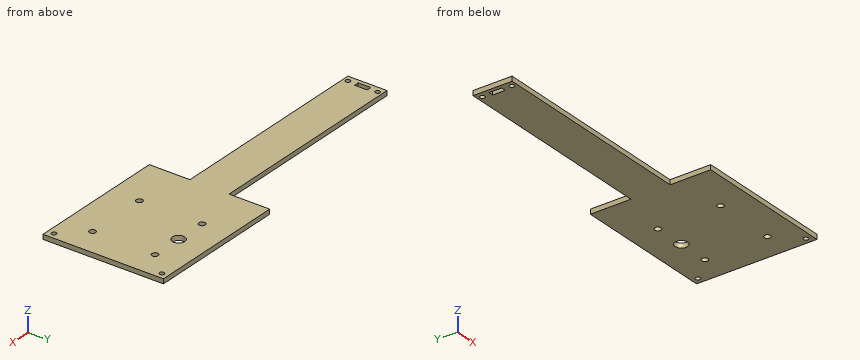
from build123d import *

# Parameters (mm, degrees)
SKETCH_1_R      = 1.5
SKETCH_1_R_2    = 2
SKETCH_1_R_3    = 4
SKETCH_1_W      = 3.1
SKETCH_1_H      = 8.1
EXTRUDE_1_DEPTH = 3


with BuildPart() as part:
    # 草图1 → 凸台-拉伸1 (new body)
    with BuildSketch(Plane.XY):
        Polygon((11.846846847, 25.617117117), (11.846846847, -51.382882883), (-78.647317431, -51.382882883), (-78.647317431, -25.382882883), (-213.153153153, -25.382882883), (-213.153153153, -0.382882883), (-78.647317431, -0.382882883), (-78.647317431, 25.617117117), align=None)
        with Locations((-209.153153153, -3.382882883)):
            Circle(SKETCH_1_R, mode=Mode.SUBTRACT)
        with Locations((7.846846847, 21.617117117)):
            Circle(SKETCH_1_R, mode=Mode.SUBTRACT)
        with Locations((-209.153153153, -22.382882883)):
            Circle(SKETCH_1_R, mode=Mode.SUBTRACT)
        with Locations((7.846846847, -47.382882883)):
            Circle(SKETCH_1_R, mode=Mode.SUBTRACT)
        with Locations((-5.653153153, -32.882882883)):
            Circle(SKETCH_1_R_2, mode=Mode.SUBTRACT)
        with Locations((-45.653153153, -32.882882883)):
            Circle(SKETCH_1_R_2, mode=Mode.SUBTRACT)
        with Locations((-45.653153153, 7.117117117)):
            Circle(SKETCH_1_R_2, mode=Mode.SUBTRACT)
        with Locations((-5.653153153, 7.117117117)):
            Circle(SKETCH_1_R_2, mode=Mode.SUBTRACT)
        with Locations((-25.653153153, 7.117117117)):
            Circle(SKETCH_1_R_3, mode=Mode.SUBTRACT)
        with Locations((-209.153153153, -12.882882883)):
            Rectangle(SKETCH_1_W, SKETCH_1_H, mode=Mode.SUBTRACT)
    extrude(amount=EXTRUDE_1_DEPTH)


solid = part.part
Design review of the part built by this model. Coordinates are the model's own, in mm. Round coordinates to 2 decimals unless told otherwise and drop trailing zeros. Order: outer loops, then holes, each group sorted by start corner. A loop starts at its lowest first (then second) coordinate and runs counter-clockwise, first axis right, second up. Notation, with made-up numbers: M -22,76.25 L 32,76.25 A30 cw 32,105.25 Z; hole C -30,0.25 d10. An arc over 180 degrees is marked long. Answer as CSV lines item,"result". Start each with the question number.
1) For pin 1 Ø0.9 at (x, z) = (-210, 2) entering from -Y; pin 2 Ø0.9 at (x, z) = (-162, 1.5) entering from +Y; pin 3 Ø1.5 at (y, z) = (10, 2) entering from -X; pin 4 Ø2.5 at (x, y) = (7.85, -47.38) entering from +Z, all flat-tipped, find the tip position at first contact; note any pin that passes through.
2) Wall thickness on line 1 along X through (y, z) = (-3.5, 0.45); line 2 along X through (y, z) = (8, 0.25); line 3 along X through (y, z) = (-34.5, 2.3): over which ranges is each line inside the solid? List them lowest first. Write a range as [from, to].
3) Add section B-B (y = -39.5). Give the boundary of the cut face in (x, z), then the cut area to 3 significant figures.
4) Add section A-A (z = 1.05). Give the number of separate pieces and of enclosed holes in the cut face, then the cut area to 3 significant figures.
5) Add section C-C (x = -85). Give the boundary of the cut face in (y, z).
Resolved:
1,pin 1,"y = -25.38"
1,pin 2,"y = -0.38"
1,pin 3,"x = -78.65"
1,pin 4,"through"
2,line 1,"[-213.15, -210.65], [-207.66, 11.85]"
2,line 2,"[-78.65, -47.45], [-43.86, -29.55], [-21.75, -7.45], [-3.86, 11.85]"
2,line 3,"[-78.65, -46.83], [-44.48, -6.83], [-4.48, 11.85]"
3,outline,"M -78.65,0 L 11.85,0 L 11.85,3 L -78.65,3 Z"
3,area,"271 mm^2"
4,separate pieces,"1"
4,enclosed holes,"10"
4,area,"10,200 mm^2"
5,outline,"M -25.38,0 L -0.38,0 L -0.38,3 L -25.38,3 Z"
